Check sheet for the modelled part. Datum: model origin and axes. Units: mm. A direction names the side the tool comes from. Give positions to 0.01 mm unless a question says otherwise; leave off trailing zeros. Write each loop counter-clockwise with the first axis right and the second up, starting at its lowest first coordinate (ties: lowest second). Pieces come first, ordered by that corner, then holes. Notation, with made-up numbers: M 63,35.25 L 94,35.25 A24 ccw 94,58.25 Z; hole C 54.5,14 d2. An arc over 180 degrees is marked long. Use CSV: the item, a comma, the result in double quotes. Start each with the question number.
1. Cross-section at B-B, the plane z = -117. Enter the section's corners in (x, y), and give its area (3 significant figures).
2. Access from +Z, -Z, +X, -X, +Y, -Y to the whole of each face (thin tool, end or side, straight path). Record for faces 1 (the face through (1, 0, -11)), 2 (the face through (-39.5, 13, -11)), 3 (the face through (-39.746, 14.915, 96.385)).
3. Cross-section at A-A, the plane x = 9. Enter the section's corners in (y, z).
4. Cross-section at C-C, the plane x = -19. Enter the section's corners in (y, z).
5. Mould release check, pull along X, two halves, no side actions. Record for faces 4 (the face through (-40, 13, -11)), 5 (the face through (6.597, 0.254, -45.865)), 6 (the face through (40, 13, -15)), 7 (the face through (1, 0.5, -11)): +X half, -X half, draft (parallel to the pull), parting line (faces both ways), or undercut.
6. Depth check by flat-ended pin: P1, Ø1, axis at x = 14, z = -65.5, coming from the +Y side; P2, Ø2.5, axis at y = 13, z = 0.47, coming from the -X side. Enter the tip coordinate at first touch or a pass-through.
7. Scan lines: line 1 (X direction, y = 6.75, z = -142); line 2 (Y direction, x = -15, z = 63). Record each from-to range of solid material in increasing order.
Autodesk Inventor part; units mm, degrees
ref_plane "YZ Plane" through (0, 0, 0) normal (1, 0, 0) x (0, 1, 0)
ref_plane "XZ Plane" through (0, 0, 0) normal (0, 1, 0) x (-1, 0, 0)
ref_plane "XY Plane" through (0, 0, 0) normal (0, 0, 1) x (1, 0, 0)
sketch "Sketch1" plane through (0, 0, 0) normal (0, 1, 0) x (-1, 0, 0)
  line L0 (40, 131.7658) -> (-40, 131.7658)
  line L1 (-40, 131.7658) -> (-40, -158.2342)
  line L2 (-40, -158.2342) -> (40, -158.2342)
  line L3 (40, -158.2342) -> (40, 131.7658)
  point P0 (0, 0)
  dimension "d0" = 80
  dimension "d1" = 290
extrude "Plate1" add sketch "Sketch1" along normal blind 0.5
sketch "Sketch2" plane through (39.5, 0, -158.2342) normal (1, 0, 0) x (0, 1, 0)
  line L0 (0, 290) -> (0, 0)
  line L1 (0, 0) -> (25, 0)
  line L2 (25, 0) -> (25, 290)
  line L3 (25, 290) -> (0, 290)
edge flange "Flange1" height 25 angle 90 thickness 0.5 bend radius 0.5 thickness toward (1, 0, 0) relief tear relief width 0.5 relief depth 0.25 edges at (40, 0.5, -13.2342) wall of the first edge with corners at (39.5, 0, 131.7658) (39.5, 0, -158.2342) (39.5, 25, -158.2342) (39.5, 25, 131.7658)
bend "Bend1"
corner "Corner1"
sketch "Sketch3" plane through (-39.5, 0, 131.7658) normal (-1, 0, 0) x (0, -1, 0)
  line L0 (0, -290) -> (0, 0)
  line L1 (0, 0) -> (-25, 0)
  line L2 (-25, 0) -> (-25, -290)
  line L3 (-25, -290) -> (0, -290)
edge flange "Flange2" height 25 angle 90 thickness 0.5 bend radius 0.5 thickness toward (-1, 0, 0) relief tear relief width 0.5 relief depth 0.25 edges at (-40, 0.5, -13.2342) wall of the first edge with corners at (-39.5, 0, -158.2342) (-39.5, 0, 131.7658) (-39.5, 25, 131.7658) (-39.5, 25, -158.2342)
bend "Bend2"
corner "Corner2"
hole "Hole1" at (9, 0, -138.2342) direction (0, 1, 0) diameter 16 depth 0.5 tip angle 118
hole "Hole2" at (9, 0, -88.2342) direction (0, 1, 0) diameter 16 depth 0.5 tip angle 118
hole "Hole3" at (9, 0, -38.2342) direction (0, 1, 0) diameter 16 depth 0.5 tip angle 118
hole "Hole4" at (9, 0, 11.7658) direction (0, 1, 0) diameter 16 depth 0.5 tip angle 118
hole "Hole5" at (9, 0, 61.7658) direction (0, 1, 0) diameter 16 depth 0.5 tip angle 118
hole "Hole6" at (9, 0, 111.7658) direction (0, 1, 0) diameter 16 depth 0.5 tip angle 118
hole "Hole7" at (-11, 0, -138.2342) direction (0, 1, 0) diameter 3 depth 0.5 tip angle 118
hole "Hole8" at (-11, 0, -88.2342) direction (0, 1, 0) diameter 3 depth 0.5 tip angle 118
hole "Hole9" at (-11, 0, -38.2342) direction (0, 1, 0) diameter 3 depth 0.5 tip angle 118
hole "Hole10" at (-11, 0, 11.7658) direction (0, 1, 0) diameter 3 depth 0.5 tip angle 118
hole "Hole11" at (-11, 0, 61.7658) direction (0, 1, 0) diameter 3 depth 0.5 tip angle 118
hole "Hole12" at (-11, 0, 111.7658) direction (0, 1, 0) diameter 3 depth 0.5 tip angle 118
hole "Hole13" at (-29, 0, -13.2342) direction (0, 1, 0) diameter 3 depth 0.5 tip angle 118
hole "Hole14" at (-29, 0, -23.2342) direction (0, 1, 0) diameter 3 depth 0.5 tip angle 118
hole "Hole15" at (-29, 0, -3.2342) direction (0, 1, 0) diameter 3 depth 0.5 tip angle 118
hole "Hole16" at (-40, 13, 91.7658) direction (1, 0, 0) diameter 10 depth 0.5 tip angle 118
hole "Hole17" at (-40, 13, 76.7658) direction (1, 0, 0) diameter 2 depth 0.5 tip angle 118
hole "Hole18" at (-40, 13, 53.7658) direction (1, 0, 0) diameter 2 depth 0.5 tip angle 118
sketch "Sketch4" plane through (-40, 25, -158.2342) normal (-1, 0, 0) x (0, 0, 1)
  line L0 (229, -15) -> (217, -15)
  line L1 (217, -15) -> (217, -9)
  line L2 (217, -9) -> (229, -9)
  line L3 (229, -9) -> (229, -15)
  line L4 (290, 0) -> (290, -24)
  point P0 (158.2342, -25)
  dimension "d185" = 61
  dimension "d186" = 73
extrude "Cut1" cut sketch "Sketch4" against normal blind 0.5
sketch "Sketch5" plane through (-40, 25, -158.2342) normal (-1, 0, 0) x (0, 0, 1)
  line L0 (198.5735, -16.892) -> (191.5735, -16.892)
  line L1 (191.5735, -16.892) -> (191.5735, -19.892)
  line L2 (191.5735, -19.892) -> (198.5735, -19.892)
  line L3 (198.5735, -19.892) -> (198.5735, -16.892)
  point P0 (158.2342, -25)
  dimension "d189" = 3
  dimension "d190" = 7
extrude "Cut2" cut sketch "Sketch5" against normal blind 0.5
hole "Hole19" at (-40, 13, 11.7658) direction (1, 0, 0) diameter 16 depth 0.5 tip angle 118
hole "Hole20" at (-40, 13, 23.0658) direction (1, 0, 0) diameter 3 depth 0.5 tip angle 118
hole "Hole21" at (-40, 13, 0.4658) direction (1, 0, 0) diameter 3 depth 0.5 tip angle 118
equation "\"d30\" = Thickness"
equation "\"d39\" = Thickness"
equation "\"d48\" = Thickness"
equation "\"d57\" = Thickness"
equation "\"d66\" = Thickness"
equation "\"d75\" = Thickness"
equation "\"d84\" = Thickness"
equation "\"d93\" = Thickness"
equation "\"d102\" = Thickness"
equation "\"d111\" = Thickness"
equation "\"d120\" = Thickness"
equation "\"d129\" = Thickness"
equation "\"d138\" = Thickness"
equation "\"d147\" = Thickness"
equation "\"d156\" = Thickness"
equation "\"d165\" = Thickness"
equation "\"d174\" = Thickness"
equation "\"d183\" = Thickness"
equation "\"d187\" = Thickness"
equation "\"d191\" = Thickness"
equation "\"d200\" = Thickness"
equation "\"d209\" = Thickness"
equation "\"d219\" = Thickness"
equation "\"d3\" = BendReliefWidth"
equation "\"d4\" = BendReliefDepth"
equation "\"d5\" = MinimumRemnant"
equation "\"d6\" = BendRadius"
equation "\"d9\" = BendRadius"
equation "\"d10\" = CornerReliefSize"
equation "\"d11\" = GapSize"
equation "\"d12\" = JacobiRadiusSize"
equation "\"d13\" = BendReliefWidth"
equation "\"d14\" = BendReliefDepth"
equation "\"d15\" = MinimumRemnant"
equation "\"d16\" = BendRadius"
equation "\"d19\" = BendRadius"
equation "\"d20\" = CornerReliefSize"
equation "\"d21\" = GapSize"
equation "\"d22\" = JacobiRadiusSize"
equation "\"BendRadius\" = Thickness"
equation "\"BendReliefWidth\" = Thickness"
equation "\"BendReliefDepth\" = 0.5 * Thickness"
equation "\"CornerReliefSize\" = 4 * Thickness"
equation "\"MinimumRemnant\" = 2 * Thickness"
equation "\"TransitionRadius\" = BendRadius"
equation "\"JacobiRadiusSize\" = BendRadius"
equation "\"GapSize\" = Thickness"
equation "\"d2\" = BendRadius"
properties part number "obudowa nowa"
Worked answers:
1,outline,"M -40,1 A1 ccw -39,0 L 39,0 A1 ccw 40,1 L 40,25 L 39.5,25 L 39.5,1 A0.5 cw 39,0.5 L -39,0.5 A0.5 cw -39.5,1 L -39.5,25 L -40,25 Z"
1,area,"64.2 mm^2"
2,face 1,"+Z, -Z, +X, -X, -Y"
2,face 2,"+Z, -Z, +Y"
2,face 3,"-X"
3,outline,"M 0,-158.23 L 0.5,-158.23 L 0.5,-146.23 L 0,-146.23 Z; M 0,-130.23 L 0.5,-130.23 L 0.5,-96.23 L 0,-96.23 Z; M 0,-80.23 L 0.5,-80.23 L 0.5,-46.23 L 0,-46.23 Z; M 0,-30.23 L 0.5,-30.23 L 0.5,3.77 L 0,3.77 Z; M 0,19.77 L 0.5,19.77 L 0.5,53.77 L 0,53.77 Z; M 0,69.77 L 0.5,69.77 L 0.5,103.77 L 0,103.77 Z; M 0,119.77 L 0.5,119.77 L 0.5,131.77 L 0,131.77 Z"
4,outline,"M 0,-158.23 L 0.5,-158.23 L 0.5,131.77 L 0,131.77 Z"
5,face 4,"-X half"
5,face 5,"undercut"
5,face 6,"+X half"
5,face 7,"undercut"
6,P1,"stops at y = 0.5"
6,P2,"stops at x = 39.5"
7,line 1,"x = -40 to -39.5, 39.5 to 40"
7,line 2,"y = 0 to 0.5"
